from build123d import *

# Parameters (mm, degrees)
F1_DEPTH  = 90
F2_W      = 64
F2_H      = 26
F3_DEPTH  = 100
F4_W      = 26
F4_H      = 26
F5_DEPTH  = 100
F6_W      = 26
F6_H      = 26
F7_DEPTH  = 105
F8_R      = 12.99999
F9_R      = 18.99999
F10_R     = 7.5
F10_R_2   = 2.5
F11_DEPTH = 25
F13_DEPTH = 25
F15_DEPTH = 25
F17_DEPTH = 25
F19_DEPTH = 25
F20_R     = 7.5
F21_DEPTH = 100


# Not quite as in the source:
# - a fillet or chamfer is up to 0.001 mm smaller than in the source, because OpenCascade refuses the exact size


with BuildPart() as f1:
    # F0 (on Front) → F1 (new body)
    with BuildSketch(Plane.XZ):
        Polygon((0, 12.5), (0, 0), (116, 0), (116, 12.5), (73.5735931288, 54.9264068712), (31.1471862576, 12.5), align=None)
    extrude(amount=F1_DEPTH)

    # F2 (on face) → F3 (cut)
    with BuildSketch(Plane(origin=(0, 0, 0), x_dir=(1, 0, 0), z_dir=(0, 0, -1))):
        with Locations((58, 77)):
            Rectangle(F2_W, F2_H)
        with Locations((58, 13)):
            Rectangle(F2_W, F2_H)
    extrude(amount=-F3_DEPTH, mode=Mode.SUBTRACT)

    # F4 (on face) → F5 (cut)
    with BuildSketch(Plane(origin=(90, 0, 0), x_dir=(0, -1, 0), z_dir=(-1, 0, 0))):
        with Locations((13, 25.5)):
            Rectangle(F4_W, F4_H)
    extrude(amount=-F5_DEPTH, mode=Mode.SUBTRACT)

    # F6 (on face) → F7 (cut)
    with BuildSketch(Plane(origin=(90, 0, 0), x_dir=(0, -1, 0), z_dir=(-1, 0, 0))):
        with Locations((77, 25.5)):
            Rectangle(F6_W, F6_H)
    extrude(amount=-F7_DEPTH, mode=Mode.SUBTRACT)

    # F8 (radius 13 in the source; OpenCascade refuses exactly that, so slightly less here)
    f8_edges = [f1.edges().sort_by_distance(p)[0] for p in [
        (0, 0, 6.25),
        (26, 0, 6.25),
        (116, -90, 6.25),
        (90, -90, 6.25),
        (26, -90, 6.25),
        (0, -90, 6.25),
        (116, 0, 6.25),
        (90, 0, 6.25),
    ]]
    fillet(f8_edges, radius=F8_R)

    # F9 (radius 19 in the source; OpenCascade refuses exactly that, so slightly less here)
    f9_edges = [f1.edges().sort_by_distance(p)[0] for p in [
        (52.36039, -64, 33.713203),
        (52.36039, -26, 33.713203),
    ]]
    fillet(f9_edges, radius=F9_R)

    # F10 (on face) → F11 (cut)
    with BuildSketch(Plane(origin=(64.25, 0, 64.25), x_dir=(0, 1, 0), z_dir=(0.7071067812, 0, 0.7071067812))):
        with Locations((-45, -38.1855518528)):
            Circle(F10_R)
        with Locations((-45, -25.6855518528)):
            Circle(F10_R_2)
        with Locations((-33.6018534744, -33.0540554063)):
            Circle(F10_R_2)
        with Locations((-56.3981465256, -33.0540554063)):
            Circle(F10_R_2)
        with Locations((-55.573814617, -44.8522185195)):
            Circle(F10_R_2)
        with Locations((-34.426185383, -44.8522185195)):
            Circle(F10_R_2)
    extrude(amount=-F11_DEPTH, mode=Mode.SUBTRACT)

    # F12 (on face) → F13 (cut)
    with BuildSketch(Plane.XY.offset(12.5)):
        with BuildLine():
            ThreePointArc((6.75, -13), (13, -19.25), (19.25, -13))
            ThreePointArc((19.25, -13), (13, -6.75), (6.75, -13))
        make_face()
        with BuildLine():
            ThreePointArc((6.75, -77), (13, -83.25), (19.25, -77))
            ThreePointArc((19.25, -77), (13, -70.75), (6.75, -77))
        make_face()
    extrude(amount=-F13_DEPTH, mode=Mode.SUBTRACT)

    # F14 (on face) → F15 (cut)
    with BuildSketch(Plane.XY.offset(12.5)):
        with BuildLine():
            ThreePointArc((96.75, -13), (103, -19.25), (109.25, -13))
            ThreePointArc((109.25, -13), (103, -6.75), (96.75, -13))
        make_face()
    extrude(amount=-F15_DEPTH, mode=Mode.SUBTRACT)

    # F16 (on face) → F17 (cut)
    with BuildSketch(Plane.XY.offset(12.5)):
        with BuildLine():
            ThreePointArc((96.75, -77), (103, -83.25), (109.25, -77))
            ThreePointArc((109.25, -77), (103, -70.75), (96.75, -77))
        make_face()
    extrude(amount=-F17_DEPTH, mode=Mode.SUBTRACT)

    # F18 (on face) → F19 (cut)
    with BuildSketch(Plane.XY.offset(12.5)):
        with BuildLine():
            Line((19.5, -38.5), (0, -38.5))
            Line((0, -38.5), (0, -45))
            Line((0, -45), (0, -51.5))
            Line((0, -51.5), (19.5, -51.5))
            ThreePointArc((19.5, -51.5), (24.0961940777, -49.5961940777), (26, -45))
            ThreePointArc((26, -45), (24.0961940777, -40.4038059223), (19.5, -38.5))
        make_face()
    extrude(amount=-F19_DEPTH, mode=Mode.SUBTRACT)

    # F20 (on face) → F21 (cut)
    with BuildSketch(Plane(origin=(64.25, 0, 64.25), x_dir=(0, 1, 0), z_dir=(0.7071067812, 0, 0.7071067812))):
        with Locations((-45, -38.1855518528)):
            Circle(F20_R)
    extrude(amount=-F21_DEPTH, mode=Mode.SUBTRACT)


solid = f1.part
The model under review builds one solid part; all positions refer to its coordinate system, in mm. A direction names the side the tool comes from. Give positions to 0.01 mm unless a question says otherwise; leave off trailing zeros. Loops run counter-clockwise (first coordinate to the right, second up) from the corner with the lowest first, then second, coordinate; pieces in that order, holes last. Notation, with made-up numbers: (19, 58) -> (45, 58) arc R17 ccw to (45, 72) -> close; hole circle Ø10 at (-24, 60). An arc over 180 degrees is marked (long way). Answer as a JSON object with one key per item and string values. Group by question number.
Q1. Take a section at A-A (y = -22). Write out the cut boundary in (x, z), plus the area to 3 significant figures.
Q2. Insertion check: pin 1 (8 mm diameter, centred on x = 17.5, z = 8, fed in from -Y); pin 2 (14.5 mm diameter, centred on x = 103, y = -13, fed in from -Z); pin 3 (7.5 mm diameter, centred on x = 13, y = -13, fed in from -Z); pin 4 (13 mm diameter, centred on x = 104, y = -8.5, fed in from +Z). Each pin has a flat end and moves straight along its axis. Give the tip position at first contact, or say it passes through.
Q3. Tool access review of faces 4 (the cylindrical face through (22.091, -86.293, 6.338)), 5 (the flat face through (10, -51.5, 6)), 6 (the flat face through (78.263, -34.461, 14.882)): name each direction out of +Z, -Z, +X, -X, +Y, -Y from which nothing blocks a thin tool from reaching the whole face with its end or side.
Q4. Draft analysis for pull direction X (two halves, no side actions). For faces 1 (the cylindrical face through (22.293, -3.909, 6.338)), 2 (the flat face through (0, -26, 6)), 3 (the cylindrical face through (112.293, -3.909, 6.338)), state which applies: pulls with the +X half, pulls with the -X half, needs draft (parallel to the pull), parting line crosses it, or undercut.
Q5. Take a section at C-C (z = 9.5). State how many separate pieces and enclosed holes the cut face has, plus the area to 3 significant figures.
Q6. Wall thickness on line 1 along Y through (x, z) = (71, 16.5); line 2 along Z through (x, y) = (24, -82.5); line 3 along X through (y, z) = (-14.5, 3.5): over which ranges is each line inside the solid? List them lowest first.
Q7. Take a section at B-B (y = -73.5). Write out the cut boundary in (x, z), plus the area to 3 significant figures.
Answer below:
{
 "1": {"outline": "(0, 0) -> (26, 0) -> (26, 12.5) -> (0, 12.5) -> close; (90, 0) -> (116, 0) -> (116, 12.5) -> (90, 12.5) -> close", "area": "650 mm2"},
 "2": {"pin 1": "stops at y = -89.99", "pin 2": "stops at z = 0", "pin 3": "passes through", "pin 4": "stops at z = 12.5"},
 "3": {"face 4": "+Z, -Z, -Y", "face 5": "+Z, -Z, -X", "face 6": "none"},
 "4": {"face 1": "undercut", "face 2": "pulls with the -X half", "face 3": "pulls with the +X half"},
 "5": {"separate pieces": "1", "enclosed holes": "5", "area": "5,760 mm2"},
 "6": {"line 1": "y = -64 to -52.49, -37.51 to -26", "line 2": "z = 0 to 12.5", "line 3": "x = 0 to 6.93, 19.07 to 26, 90 to 96.93, 109.07 to 116"},
 "7": {"outline": "(0, 0) -> (7.82, 0) -> (7.82, 12.5) -> (0, 12.5) -> close; (18.18, 0) -> (26, 0) -> (26, 12.5) -> (18.18, 12.5) -> close; (90, 0) -> (97.82, 0) -> (97.82, 12.5) -> (90, 12.5) -> close; (108.18, 0) -> (116, 0) -> (116, 12.5) -> (108.18, 12.5) -> close", "area": "391 mm2"}
}
